from build123d import *

# Parameters (mm, degrees)
F0_R          = 5.28
F1_DEPTH      = 16
F2_R          = 2.28
F3_DEPTH      = 2.25
F4_R          = 4.25
F5_DEPTH      = 25
F5_DEPTH_BACK = 3


with BuildPart() as f1:
    # F0 (on Front) → F1 (new body)
    with BuildSketch(Plane.XZ):
        Circle(F0_R)
    extrude(amount=F1_DEPTH)

    # F2 (on face) → F3 (cut)
    with BuildSketch(Plane.XZ.offset(16)):
        Circle(F2_R)
    extrude(amount=-F3_DEPTH, mode=Mode.SUBTRACT)

    # F4 (on Top) → F5 (cut, two sides)
    with BuildSketch(Plane.XY) as f5_sk:
        with Locations((0, -5)):
            Circle(F4_R)
    extrude(amount=-F5_DEPTH, mode=Mode.SUBTRACT)
    extrude(f5_sk.sketch, amount=F5_DEPTH_BACK, mode=Mode.SUBTRACT)


solid = f1.part
Geometry: final body of the model. Coordinates: model frame, mm. A direction names the side the tool comes from. Give positions to 0.01 mm unless a question says otherwise; leave off trailing zeros. Write each loop counter-clockwise with the first axis right and the second up, starting at its lowest first coordinate (ties: lowest second). Pieces come first, ordered by that corner, then holes. Notation, with made-up numbers: (-27, -4) -> (-16, -4) arc R12 cw to (-16, 2) -> close; hole circle Ø1 at (48.25, 69). An arc over 180 degrees is marked (long way). Answer as a JSON object with one key per item and string values.
1. Cut plane D-D on z = 4. Output: boundary loops of the cut face in (x, y), and give its area (3 significant figures).
Ans:
{"outline": "(-3.45, -16) -> (3.45, -16) -> (3.45, 0) -> (-3.45, 0) -> close", "area": "110 mm^2"}
2. Mould query, pull axis X, two halves, no side actions, for faces 4 (the cylindrical face through (-0.687, -7.888, 5.235)), 5 (the flat face through (2.3, -16, -1.1)), 6 (the flat face through (0, -13.75, 0)). Classes: pulls with the +X half, pulls with the -X half, needs draft (parallel to the pull), parting line crosses it, or undercut.
Ans:
{"face 4": "parting line crosses it", "face 5": "needs draft", "face 6": "undercut"}
3. Cut plane C-C on y = -4.25. Output: boundary loops of the cut face in (x, z), and give its area (3 significant figures).
Ans:
{"outline": "(-4.18, -3.22) -> (-4.18, 3) -> (4.18, 3) -> (4.18, -3.22) arc R5.28 ccw (long way) to start", "area": "23.5 mm^2"}
4. Ray query, probe 1 along Z at (x, y) = (0, -15.25); probe 2 along Y at (x, z) = (0, -4); probe 3 along Y at (x, z) = (0, 0). Return the intervals inside material, ascending. Write a range as from..to.
Ans:
{"probe 1": "z = -5.28..-2.28, 2.28..5.28", "probe 2": "y = -16..-9.25, -0.75..0", "probe 3": "y = -13.75..-9.25, -0.75..0"}
5. Contact query for flat-ended pins moving along their axis: pin 1 (3.5 mm diameter, centred on x = 0, z = -0.5, fed in from -Y); pin 2 (5 mm diameter, centred on x = -0.5, y = -11.5, fed in from -Z); pin 3 (4 mm diameter, centred on y = -7.5, z = 4, fed in from +X); pin 4 (1 mm diameter, centred on x = 4, y = -9.5, fed in from -Z). Output: stop coordinate, or through.
Ans:
{"pin 1": "stops at y = -13.75", "pin 2": "stops at z = -5.28", "pin 3": "stops at x = 4.89", "pin 4": "stops at z = -3.95"}
6. Access query for faces 1 (the cylindrical face through (-1.8, -14.9, -1.4)), 2 (the flat face through (0, -5, 3)), 3 (the flat face through (0, 0, 0)). Directions: +Z, -Z, +X, -X, +Y, -Y. A direction counts if a zero-diameter tool reaches every point of the face in a straight line with its end or side. Return the directions, or none.
Ans:
{"face 1": "-Y", "face 2": "-Z", "face 3": "+Z, -Z, +X, -X, +Y"}
7. Cut plane A-A on x = 0. Output: boundary loops of the cut face in (y, z), and give its area (3 significant figures).
Ans:
{"outline": "(-16, -5.28) -> (-9.25, -5.28) -> (-9.25, 3) -> (-0.75, 3) -> (-0.75, -5.28) -> (0, -5.28) -> (0, 5.28) -> (-16, 5.28) -> (-16, 2.28) -> (-13.75, 2.28) -> (-13.75, -2.28) -> (-16, -2.28) -> close", "area": "88.3 mm^2"}
8. Cut plane B-B on z = 2. Output: boundary loops of the cut face in (x, y).
Ans:
{"outline": "(-4.89, -16) -> (-1.09, -16) -> (-1.09, -13.75) -> (1.09, -13.75) -> (1.09, -16) -> (4.89, -16) -> (4.89, 0) -> (-4.89, 0) -> close; hole circle Ø8.5 at (0, -5)"}
